Geometry check sheet. Reference: drawing and pictorial views, mm from the part's lowest x, y, z. A direction names the side the tool comes from. Round coordinates to 2 decimals unless told otherwise and drop trailing zeros. Order: outer loops, then holes, each group sorted by start corner. A loop starts at its lowest first (then second) coordinate and runs counter-clockwise, first axis right, second up.
(1) Release check for a two-part mould opening along Y. For the marked faces 4, 5, 6 and 7 record: +Y half, -Y half, draft (parallel to the pull), parting line (faces both ways), or undercut.
(2) Sectioned sample at A-A (x = 3.5). Give the number of separate pieces and of enclosed holes in the cut face, plus the area to 3 significant figures.
(3) Set-up check for the marked faces 1, 2 and 3: record each of +Z, -Z, +X, -X, +Y, -Y from which the full face is reachable in a straight line by a thin tool's end or side.
(4) Sectioned sample at C-C (y = 27). Record the boundary of the cut face in (x, z).
(5) Sectioned sample at D-D (z = 5.75). Record the boundary of the cut face in (x, y).
(6) Material ranges on line 1 along Y through (x, z) = (3.5, 3.35); line 2 along Y through (x, z) = (3.5, 4.25); line 3 along Z through (x, y) = (0.75, 36), recorded low to high.
(7) Go/stop test with flat-tipped pins: pin 1 (1.5 mm diameter, centred on x = 3.5, z = 2, fed in from -Y); pin 2 (2 mm diameter, centred on y = 5, z = 4, fed in from -X); pin 3 (3 mm diameter, centred on x = 5.5, y = 29.5, fed in from +Z). Record where each tip stops, or that it passes through.
(8) Sectioned sample at B-B (z = 4). Record the boundary of the cut face in (x, y).
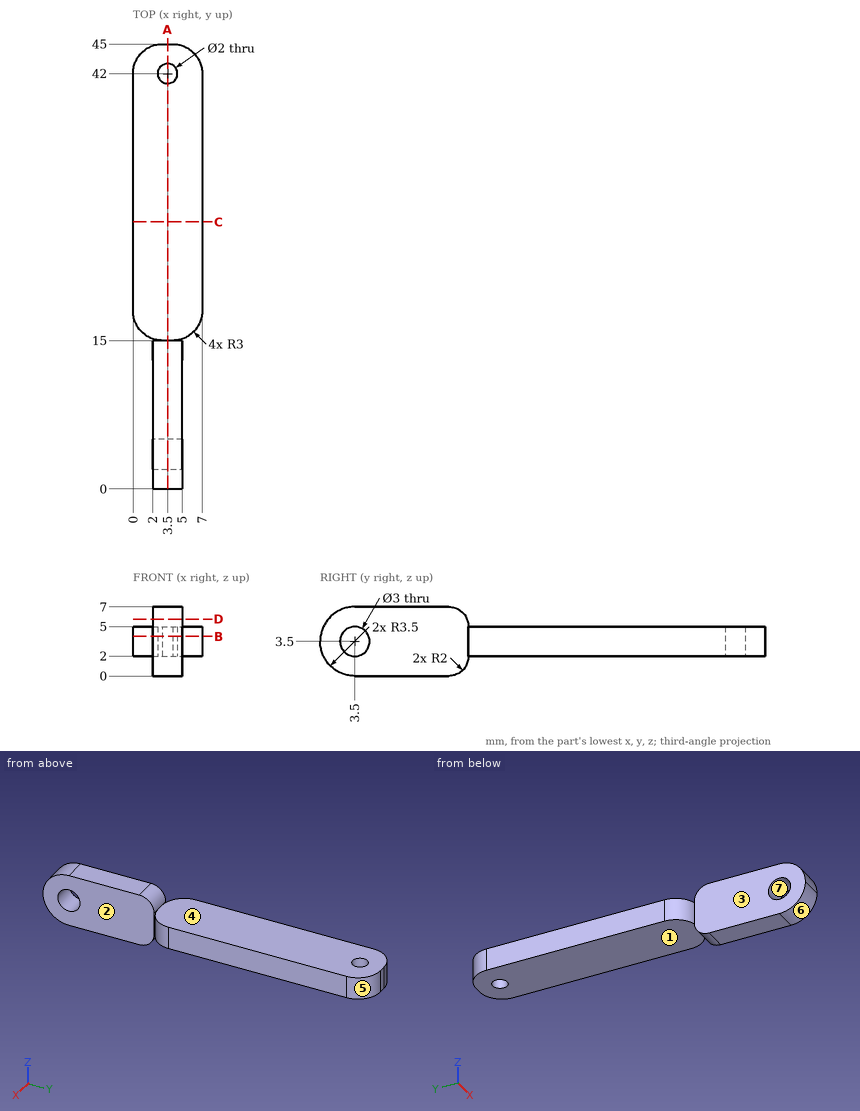
Answer below:
1. face 4: draft
1. face 5: +Y half
1. face 6: -Y half
1. face 7: undercut
2. separate pieces: 2
2. enclosed holes: 1
2. area: 175 mm2
3. face 1: -Z, +X, -X, +Y
3. face 2: +Z, -Z, +X, -Y
3. face 3: +Z, -Z, -X, -Y
4. outline: (0, 2) - (7, 2) - (7, 5) - (0, 5) - close
5. outline: (2, 0.82) - (5, 0.82) - (5, 14.85) - (2, 14.85) - close
6. line 1: y = 0 to 2.01, 4.99 to 41, 43 to 45
6. line 2: y = 0.08 to 2.2, 4.8 to 41, 43 to 45
6. line 3: z = 2 to 5
7. pin 1: stops at y = 0.08
7. pin 2: stops at x = 2
7. pin 3: stops at z = 5
8. outline: (0, 18) arc R3 ccw to (3, 15) - (2, 15) - (2, 4.91) - (5, 4.91) - (5, 15) - (4, 15) arc R3 ccw to (7, 18) - (7, 42) arc R3 ccw to (4, 45) - (3, 45) arc R3 ccw to (0, 42) - close; (2, 0.04) - (5, 0.04) - (5, 2.09) - (2, 2.09) - close; hole circle Ø2 at (3.5, 42)
